Solid Edge part; units mm, degrees
sketch "Sketch1" plane through (0, 0, 0) normal (0, 0, 1) x (1, 0, 0)
  line L0 (-8.5, -7.5) -> (8.5, -7.5)
  line L1 (8.5, -7.5) -> (8.5, 7.5)
  line L2 (8.5, 7.5) -> (-8.5, 7.5)
  line L3 (-8.5, 7.5) -> (-8.5, -7.5)
  dimension "D1" = 8.5
  dimension "D2" = 8.5
extrude "Protrusion1" add sketch "Sketch1" along normal blind 3
fillet "Verrundung_1" radius 7 2 edges at (-8.5, -7.5, 1.5) (-8.5, 7.5, 1.5)
hole "Bohrung_1" at (5, 0, 3) direction (0, 0, -1) diameter 3.6 depth 3 countersink diameter 6.5 countersink angle 90
sketch "Sketch2" plane through (0, 0, 0) normal (0, 0, -1) x (1, 0, 0)
  circle A0 centre (1, 4.5) radius 1.25
extrude "v_3" add sketch "Sketch2" along normal blind 3
fillet "Verrundung_2" radius 0.2 1 edges at (-0.25, -4.5, -3)
fillet "Verrundung_3" radius 0.2 14 edges at (-6.4497, -5.4497, 3) (3.5, -7.5, 3) (-8.5, 0, 3) (-6.4497, 5.4497, 3) (3.5, 7.5, 3) (8.5, 0, 3) (8.5, -7.5, 1.5) (8.5, 7.5, 1.5) (-6.4497, -5.4497, 0) (-8.5, 0, 0) (-6.4497, 5.4497, 0) (3.5, 7.5, 0) (3.5, -7.5, 0) (8.5, 0, 0)
For this review, take the finished solid that the model builds, in its own axes (mm). A direction names the side the tool comes from. Round coordinates to 2 decimals unless told otherwise and drop trailing zeros. Order: outer loops, then holes, each group sorted by start corner. A loop starts at its lowest first (then second) coordinate and runs counter-clockwise, first axis right, second up.
Q1. We need section B-B, the plane z = 1.2. Give the boundary of the cut face in (x, y), plus the area to 3 significant figures.
Findings below:
outline: (-8.5, -0.5) arc R7 ccw to (-1.5, -7.5) - (8.3, -7.5) arc R0.2 ccw to (8.5, -7.3) - (8.5, 7.3) arc R0.2 ccw to (8.3, 7.5) - (-1.5, 7.5) arc R7 ccw to (-8.5, 0.5) - close; hole circle Ø3.6 at (5, 0)
area: 224 mm2
Q2. Mouldability with a two-part tool opening along X and no side actions: class faces 1 (the flat face through (0, 0, 0)), 2 (the flat face through (-8.5, 0, 1)), 3 (the cylindrical face through (3.215, 0.234, 0.764)), 4 (the flat face through (8.5, 0, 1)) as pulls with the +X half, pulls with the -X half, needs draft (parallel to the pull), parting line crosses it, or undercut.
Findings below:
face 1: needs draft
face 2: pulls with the -X half
face 3: undercut
face 4: pulls with the +X half
Q3. We need section A-A, the plane y = 0. Give the boundary of the cut face in (x, z), plus the area to 3 significant figures.
Findings below:
outline: (-8.5, 0.2) arc R0.2 ccw to (-8.3, 0) - (3.2, 0) - (3.2, 1.55) - (1.75, 3) - (-8.3, 3) arc R0.2 ccw to (-8.5, 2.8) - close; (6.8, 0) - (8.3, 0) arc R0.2 ccw to (8.5, 0.2) - (8.5, 2.8) arc R0.2 ccw to (8.3, 3) - (8.25, 3) - (6.8, 1.55) - close
area: 38.1 mm2
Q4. Wall thickness on line 1 (Y direction, x = 5, z = 0.95); line 2 (Z direction, x = 1.5, y = 0.5); line 3 (Y direction, x = 5, z = 2.7): over which ranges is each line inside the solid? List them lowest first.
Findings below:
line 1: y = -7.5 to -1.8, 1.8 to 7.5
line 2: z = 0 to 3
line 3: y = -7.5 to -2.95, 2.95 to 7.5
Q5. We need section C-C, the plane x = 1. Give the boundary of the cut face in (y, z).
Findings below:
outline: (-7.5, 0.2) arc R0.2 ccw to (-7.3, 0) - (-5.75, 0) - (-5.75, -2.8) arc R0.2 ccw to (-5.55, -3) - (-3.45, -3) arc R0.2 ccw to (-3.25, -2.8) - (-3.25, 0) - (7.3, 0) arc R0.2 ccw to (7.5, 0.2) - (7.5, 2.8) arc R0.2 ccw to (7.3, 3) - (-7.3, 3) arc R0.2 ccw to (-7.5, 2.8) - close
Q6. Machinability: for faces 5 (the flat face through (3, -7.5, 1)), 6 (the cylindrical face through (0.73, -5.72, -1.38)), which of the approach directions +Z, -Z, +X, -X, +Y, -Y give a long, thin tool a straight path to every point of the face, cutting with its end or side? Answer none if there is none.
Findings below:
face 5: +Z, -Z, +X, -X, -Y
face 6: -Z
Q7. We need section D-D, the plane z = -1.4. Give the boundary of the cut face in (x, y).
Findings below:
outline: circle Ø2.5 at (1, -4.5)
Q8. Insertion check: P1, Ø3, axis at x = 5, y = 0, coming from the +Z side; P2, Ø3, axis at y = -4.5, z = -2, coming from the +X side. Each pin has a flat end and moves straight along its axis. Give the tip position at first contact, or say it passes through.
Findings below:
P1: passes through
P2: stops at x = 2.25
